Source: three-view drawing plus pictorial views. Frame: mm from the lowest corner of the part. Give positions to 0.01 mm unless a question says otherwise; leave off trailing zeros. Loops run counter-clockwise (first coordinate to the right, second up) from the corner with the lowest first, then second, coordinate; pieces in that order, holes last.
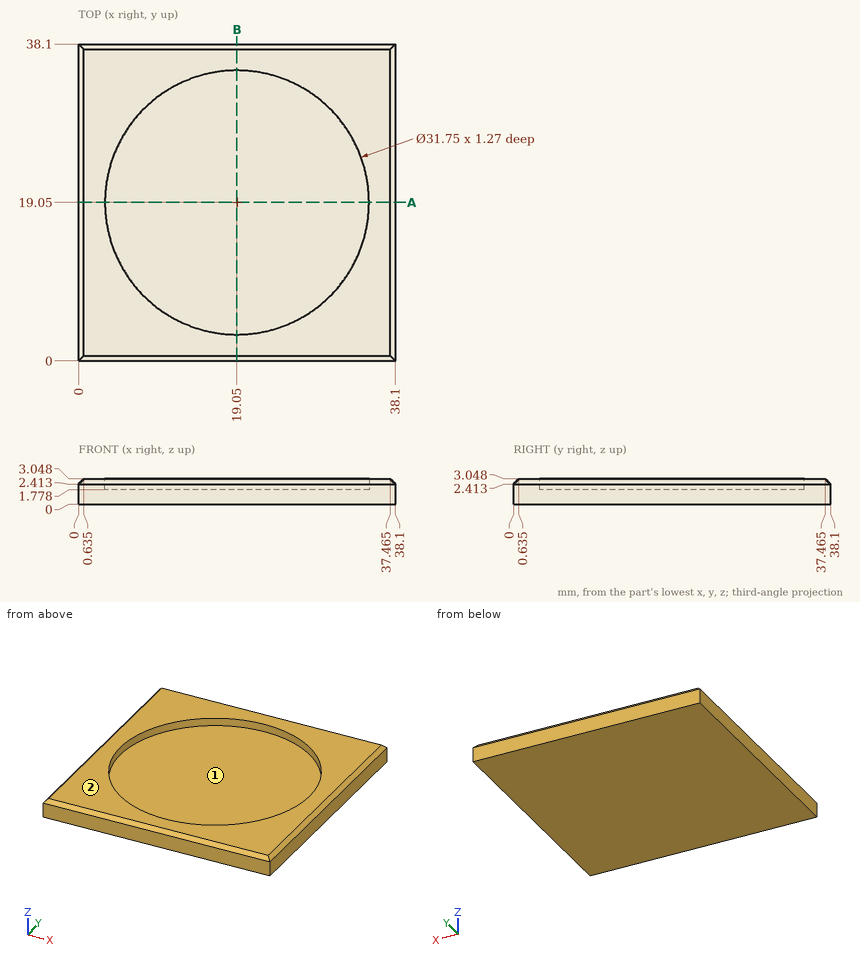
1) Cut plane A-A (y = 19.05). Return loops of the section in (x, z) (3 decimals).
Checks:
outline: (0, 0) - (38.1, 0) - (38.1, 2.413) - (37.465, 3.048) - (34.925, 3.048) - (34.925, 1.778) - (3.175, 1.778) - (3.175, 3.048) - (0.635, 3.048) - (0, 2.413) - close
2) Ray query, probe 1 along Y at (x, z) = (19.05, 2.15) (3 decimals); probe 2 along Z at (x, y) = (21, 7); probe 3 along X at (y, z) = (31, 2.8). Return the intervals inside material, ascending.
Checks:
probe 1: y = 0 to 3.175, 34.925 to 38.1
probe 2: z = 0 to 1.78
probe 3: x = 0.39 to 8.6, 29.5 to 37.71
3) Pull-direction query (Y, two-part tool) for the marked faces 1 and 2; classes: released by +Y, released by -Y, zero draft, split by the parting line, or undercut.
Checks:
face 1: undercut
face 2: zero draft
4) Contact query for a flat-ended pin moving along its axis: P1, Ø9.5, axis at x = 18, y = 23.5, coming from the +Z side. Output: stop coordinate, or through.
Checks:
P1: stops at z = 1.78
